```python
from build123d import *

# Parameters (mm, degrees)
SKETCH1_W           = 105
SKETCH1_H           = 105
BOSS_EXTRUDE1_DEPTH = 50
CUT_EXTRUDE1_DEPTH  = 106
SKETCH3_W           = 90
SKETCH3_H           = 90
CUT_EXTRUDE2_DEPTH  = 18
SKETCH4_W           = 50
SKETCH4_H           = 30
CUT_EXTRUDE3_DEPTH  = 9
SKETCH5_W           = 3
SKETCH5_H           = 50
CUT_EXTRUDE4_DEPTH  = 106
SKETCH7_W           = 12
SKETCH7_H           = 14
CUT_EXTRUDE5_DEPTH  = 5


with BuildPart() as part:
    # Sketch1 → Boss-Extrude1 (new body)
    with BuildSketch(Plane.XY):
        Rectangle(SKETCH1_W, SKETCH1_H)
    extrude(amount=BOSS_EXTRUDE1_DEPTH)

    # Sketch2 → Cut-Extrude1 (cut, through all)
    with BuildSketch(Plane.XZ.offset(52.5)):
        with BuildLine():
            Line((-42.5, 8), (-42.5, 0))
            Line((-42.5, 0), (42.5, 0))
            Line((42.5, 0), (42.5, 8))
            ThreePointArc((42.5, 8), (0, 17.480665049), (-42.5, 8))
        make_face()
    extrude(amount=-CUT_EXTRUDE1_DEPTH, mode=Mode.SUBTRACT)

    # Sketch3 → Cut-Extrude2 (cut)
    with BuildSketch(Plane.XY.offset(50)):
        Rectangle(SKETCH3_W, SKETCH3_H)
    extrude(amount=-CUT_EXTRUDE2_DEPTH, mode=Mode.SUBTRACT)

    # Sketch4 → Cut-Extrude3 (cut)
    with BuildSketch(Plane.XY.offset(32)):
        Rectangle(SKETCH4_W, SKETCH4_H)
    extrude(amount=-CUT_EXTRUDE3_DEPTH, mode=Mode.SUBTRACT)

    # Sketch5 → Cut-Extrude4 (cut, through all)
    with BuildSketch(Plane.ZY.offset(52.5)):
        with Locations((4.5, 0)):
            Rectangle(SKETCH5_W, SKETCH5_H)
    extrude(amount=-CUT_EXTRUDE4_DEPTH, mode=Mode.SUBTRACT)

    # Sketch7 → Cut-Extrude5 (cut)
    with BuildSketch(Plane(origin=(52.5, 0, 0), x_dir=(0, 0, -1), z_dir=(1, 0, 0))):
        with Locations((-40, 2.495495841)):
            Rectangle(SKETCH7_W, SKETCH7_H)
    extrude(amount=-CUT_EXTRUDE5_DEPTH, mode=Mode.SUBTRACT)


solid = part.part
```
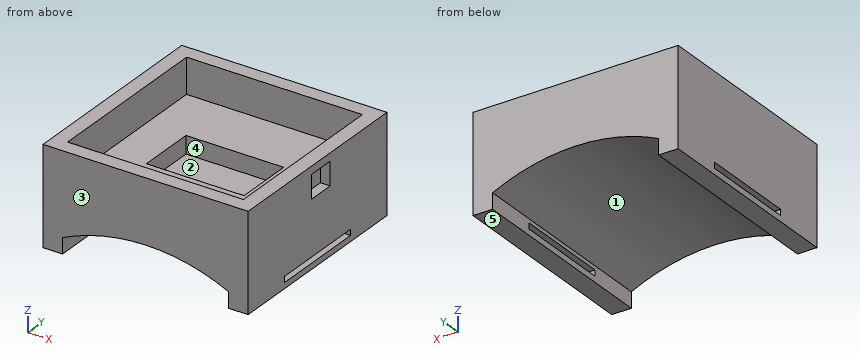
Can you work these out from the model? Positions are in its coordinate system, mm. Face numbers are marked on the shaded views. A direction names the side the tool comes from. Coordinates: 2 decimals unless noted, no trailing zeros. Loops run counter-clockwise (first coordinate to the right, second up) from the corner with the lowest first, then second, coordinate; pieces in that order, holes last.
1) Imagine slicing it at B-B on z = 29.5. List the corners of the cut face in (x, y) for me, plus the area to 4 significant figures.
2) For pin 1 (3 mm diameter, centred on x = 22, y = -31, fed in from +Z); pin 2 (3 mm diameter, centred on x = 10, y = 0.5, fed in from +Z); pin 3 (10 mm diameter, centred on x = -27.5, y = -33.5, fed in from -Z), each with a flat end and sliding along its axis, tell me the tip position at first contact or that it passes through.
3) Imagine slicing it at C-C on y = 38. List the corners of the cut face in (x, z) for me, plus the area to 3 significant figures.
4) Which directions (+Z, -Z, +X, -X, +Y, -Y) give clear straight access to the entire face, cutting with the end or side of a thin tool? Please do the marked faces 4 and 5.
5) I need wall thicknesses on probe 1 along Y at (x, z) = (14, 24); probe 2 along Z at (x, y) = (-47, 7); probe 3 along X at (y, z) = (-13, 8). Which ranges of each line are inside material? Lowest first, please.
6) Thinking about a two-plate mould opening in Y: for the marked faces 1, 2 and 3, which applies, pulls with the +Y half, pulls with the -Y half, needs draft (parallel to the pull), parting line crosses it, or undercut?
7) Imagine slicing it at A-A on y = -8. List the corners of the cut face in (x, z) for me.
8) Imagine slicing it at D-D on z = 11. List the corners of the cut face in (x, y) for me, plus the area to 3 significant figures.
Completed:
1. outline: (-52.5, -52.5) - (52.5, -52.5) - (52.5, 52.5) - (-52.5, 52.5) - close; hole (-25, -15) - (25, -15) - (25, 15) - (-25, 15) - close
1. area: 9,525 mm2
2. pin 1: stops at z = 32
2. pin 2: stops at z = 23
2. pin 3: stops at z = 12.05
3. outline: (-52.5, 0) - (-42.5, 0) - (-42.5, 8) arc R100 cw to (42.5, 8) - (42.5, 0) - (52.5, 0) - (52.5, 50) - (45, 50) - (45, 32) - (-45, 32) - (-45, 50) - (-52.5, 50) - close
3. area: 2,410 mm2
4. face 4: +Z
4. face 5: -Z, +X, -X, +Y, -Y
5. probe 1: y = -52.5 to -15, 15 to 52.5
5. probe 2: z = 0 to 3, 6 to 50
5. probe 3: x = -52.5 to -42.5, 42.5 to 52.5
6. face 1: needs draft
6. face 2: undercut
6. face 3: pulls with the -Y half
7. outline: (-52.5, 0) - (-42.5, 0) - (-42.5, 3) - (-52.5, 3) - close; (-52.5, 6) - (-42.5, 6) - (-42.5, 8) arc R100 cw to (42.5, 8) - (42.5, 6) - (52.5, 6) - (52.5, 50) - (45, 50) - (45, 32) - (25, 32) - (25, 23) - (-25, 23) - (-25, 32) - (-45, 32) - (-45, 50) - (-52.5, 50) - close; (42.5, 0) - (52.5, 0) - (52.5, 3) - (42.5, 3) - close
8. outline: (-52.5, -52.5) - (-35.41, -52.5) - (-35.41, 52.5) - (-52.5, 52.5) - close; (35.41, -52.5) - (52.5, -52.5) - (52.5, 52.5) - (35.41, 52.5) - close
8. area: 3,590 mm2
